Job drawing, mm, ordinate dimensions from the low corner. One solid piece. Give positions to 0.01 mm unless a question says otherwise; leave off trailing zeros. Order: outer loops, then holes, each group sorted by start corner. A loop starts at its lowest first (then second) coordinate and runs counter-clockwise, first axis right, second up. Notation, with made-up numbers: (-8, 54) -> (42, 54) arc R18 cw to (42, 68) -> close; hole circle Ø11 at (48, -28). An arc over 180 degrees is marked (long way). Write item = value, one per line. Start each with the question number.
(1) Saw through at D-D, the plane x = 76. List the corners of the cut face in (y, z) (1 decimal).
(2) Saw through at C-C, the plane x = 50.5. List the corners of the cut face in (y, z) (1 decimal), then the cut area to 3 significant figures.
(3) Probe line 1 along X through (y, z) = (13.5, 8.5) (1 decimal); line 2 along Y through (x, z) = (59, 2.5) (1 decimal); line 3 along X through (y, z) = (27, 0.5). List the from-to ranges inside material, lowest first. Write a range as from..to.
(4) Two-plate mould, pull along X, no slides. Class the marked faces 1, 2, 3 and 4: pulls with the +X half, pulls with the -X half, needs draft (parallel to the pull), parting line crosses it, or undercut.
(5) Saw through at B-B, the plane z = 4.75. List the corners of the cut face in (x, y) (1 decimal).
(6) Flat gauge pin, fed straight in: pin 1 (11.5 mm diameter, centred on x = 38, y = 34, fed in from +Z). Where does the tip first touch, or does it go through?
(7) Saw through at A-A, the plane y = 43. List the corners of the cut face in (x, z) (1 decimal), then the cut area to 3 significant figures.
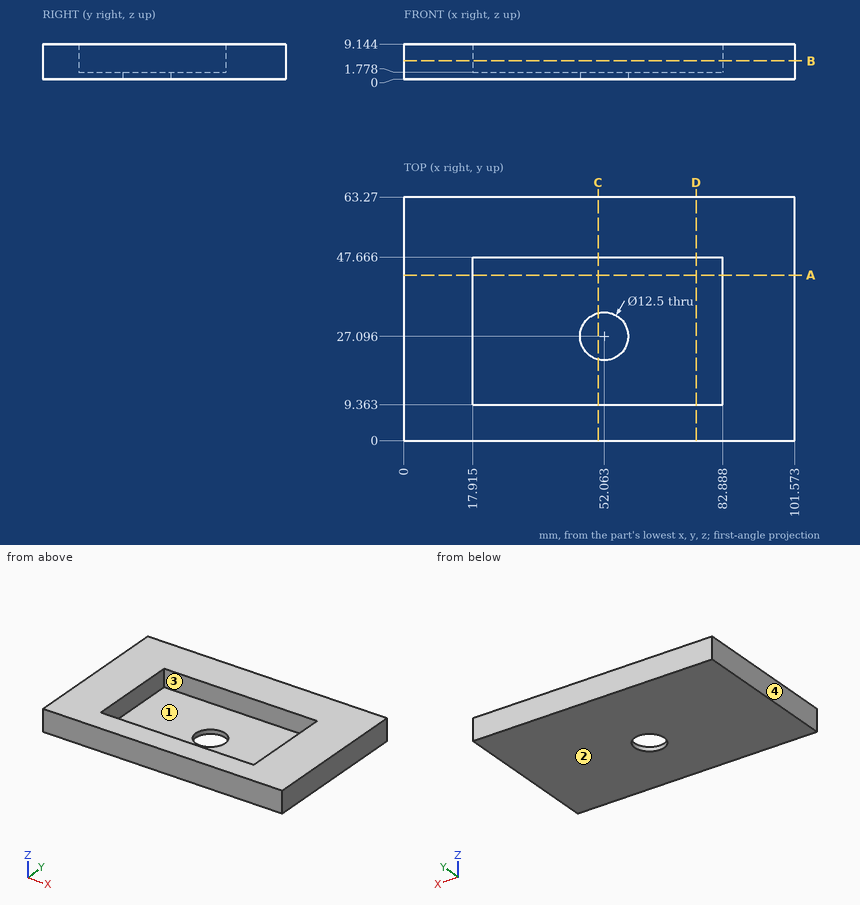
Results list:
q1.outline = (0, 0) -> (63.3, 0) -> (63.3, 9.1) -> (47.7, 9.1) -> (47.7, 1.8) -> (9.4, 1.8) -> (9.4, 9.1) -> (0, 9.1) -> close
q2.outline = (0, 0) -> (21, 0) -> (21, 1.8) -> (9.4, 1.8) -> (9.4, 9.1) -> (0, 9.1) -> close; (33.1, 0) -> (63.3, 0) -> (63.3, 9.1) -> (47.7, 9.1) -> (47.7, 1.8) -> (33.1, 1.8) -> close
q2.area = 275 mm^2
q3.line_1 = 0..17.9, 82.9..101.6
q3.line_2 = 0..9.4, 47.7..63.3
q3.line_3 = 0..45.81, 58.31..101.57
q4.face_1 = undercut
q4.face_2 = needs draft
q4.face_3 = undercut
q4.face_4 = pulls with the -X half
q5.outline = (0, 0) -> (101.6, 0) -> (101.6, 63.3) -> (0, 63.3) -> close; hole (17.9, 9.4) -> (82.9, 9.4) -> (82.9, 47.7) -> (17.9, 47.7) -> close
q6.pin_1 = 1.78
q7.outline = (0, 0) -> (101.6, 0) -> (101.6, 9.1) -> (82.9, 9.1) -> (82.9, 1.8) -> (17.9, 1.8) -> (17.9, 9.1) -> (0, 9.1) -> close
q7.area = 450 mm^2
